Autodesk Inventor part; units mm, degrees
ref_plane "YZ Plane" through (0, 0, 0) normal (1, 0, 0) x (0, 1, 0)
ref_plane "XZ Plane" through (0, 0, 0) normal (0, 1, 0) x (-1, 0, 0)
ref_plane "XY Plane" through (0, 0, 0) normal (0, 0, 1) x (1, 0, 0)
sketch "Skizze1" plane through (0, 0, 0) normal (0, 0, 1) x (1, 0, 0)
  line L0 (-52.5, -10.25) -> (52.5, -10.25)
  line L1 (52.5, -10.25) -> (52.5, 10.25)
  line L2 (52.5, 10.25) -> (-52.5, 10.25)
  line L3 (-52.5, 10.25) -> (-52.5, -10.25)
  line L4 (-52.5, -10.25) -> (52.5, 10.25) construction
  line L5 (52.5, -10.25) -> (-52.5, 10.25) construction
  line L6 (-52.5, 0) -> (52.5, 0) construction
  circle A0 centre (-22.5, 0) radius 2.75
  circle A1 centre (22.5, 0) radius 2.75
  line L7 (0, -14.35) -> (0, 14.35) construction
  point P0 (0, 0)
  dimension "d0" = 105
  dimension "d1" = 20.5
  dimension "d2" = 5.5
  dimension "d3" = 5.5
  dimension "d4" = 45
sketch "Skizze2" plane through (0, 0, 0) normal (1, 0, 0) x (0, 1, 0)
  line L0 (-14.35, 0) -> (14.35, 0) construction
  line L1 (0.25, 0) -> (10.25, 0)
  line L2 (10.25, 0) -> (10.25, 20.5)
  line L3 (10.25, 20.5) -> (0.25, 20.5)
  line L4 (0.25, 20.5) -> (0.25, 0)
  line L5 (0.25, 0) -> (7.85, 0)
  line L6 (7.85, 0) -> (7.85, 18.1)
  line L7 (7.85, 18.1) -> (0.25, 18.1)
  line L8 (0.25, 18.1) -> (0.25, 0)
  point P0 (0, 0)
  point P1 (10.25, 0)
  point P2 (0.25, 18.1)
  dimension "d5" = 20.5
  dimension "d6" = 2.4
  dimension "d7" = 2.4
  dimension "d12" = 10
extrude "Extrusion1" add sketch "Skizze1" against normal blind 1.8
extrude "Extrusion2" add sketch "Skizze2" along normal mid plane 105 contours L6 L7 L4 L3 L2 L1
equation "\"d7\" = d6"
equation "\"d10\" = d0"
properties part number "Door_Handle" material "ABS-Kunststoff"
Here's how the part is built. I have some questions about the finished solid (model axes, mm). A direction names the side the tool comes from. Coordinates: 2 decimals unless noted, no trailing zeros. Write each loop counter-clockwise with the first axis right and the second up, starting at its lowest first coordinate (ties: lowest second). Pieces come first, ordered by that corner, then holes. Notation, with made-up numbers: (50.25, 72.25) - (97.25, 72.25) arc R20 cw to (97.25, 105.25) - close; hole circle Ø2 at (-21.75, -17). An arc over 180 degrees is marked (long way). Use one line per item in the form item = value.
1) Suppose I cut it at C-C, the plane z = 5.5. Write out the boundary of the cut face in (x, y), plus the area to 3 significant figures.
Solved:
outline = (-52.5, 7.85) - (52.5, 7.85) - (52.5, 10.25) - (-52.5, 10.25) - close
area = 252 mm2
2) Thinking about a two-plate mould opening in Z: for faces 1 (the flat face through (-1, 0, -1.8)), 2 (the flat face through (-1, 4, 18.1)), 3 (the flat face through (-1, 0.25, 19)), which applies, released by +Z, released by -Z, zero draft, split by the parting line, or undercut?
Solved:
face_1 = released by -Z
face_2 = undercut
face_3 = zero draft
3) On a 3-axis mill with a long thin cutter (end or side, diameter ignored), from which of +Z, -Z, +X, -X, +Y, -Y can I reach the whole of each face in a straight line? I mean faces 4 (the flat face through (-52.5, 8, 8)), 5 (the flat face through (-1, -1, 0)), 6 (the cylindrical face through (-25.247, 0.121, -0.887)). Say none if no direction works.
Solved:
face_4 = +Z, -Z, -X, +Y, -Y
face_5 = +X, -X, -Y
face_6 = -Z
4) I need wall thicknesses on line 1 (Y direction, x = -22.5, z = -0.8); line 2 (Z direction, x = -27.5, y = 2.25); line 3 (Y direction, x = 33.5, z = 14.25). Which ranges of each line are inside material? Lowest first, please.
Solved:
line_1 = -10.25 to -2.75, 2.75 to 10.25
line_2 = -1.8 to 0, 18.1 to 20.5
line_3 = 7.85 to 10.25
5) Suppose I cut it at D-D, the plane y = -8.5. Write out the boundary of the cut face in (x, z), plus the area to 3 significant figures.
Solved:
outline = (-52.5, -1.8) - (52.5, -1.8) - (52.5, 0) - (-52.5, 0) - close
area = 189 mm2
6) Suppose I cut it at B-B, the plane y = 6.25. Write out the boundary of the cut face in (x, z), plus the area to 3 significant figures.
Solved:
outline = (-52.5, -1.8) - (52.5, -1.8) - (52.5, 0) - (-52.5, 0) - close; (-52.5, 18.1) - (52.5, 18.1) - (52.5, 20.5) - (-52.5, 20.5) - close
area = 441 mm2
7) Suppose I cut it at A-A, the plane x = -22.5. Write out the boundary of the cut face in (y, z).
Solved:
outline = (-10.25, -1.8) - (-2.75, -1.8) - (-2.75, 0) - (-10.25, 0) - close; (0.25, 18.1) - (7.85, 18.1) - (7.85, 0) - (2.75, 0) - (2.75, -1.8) - (10.25, -1.8) - (10.25, 20.5) - (0.25, 20.5) - close
8) I'm going to push flat-ended pins straight in: P1, Ø2, axis at y = -1, z = 18, coming from the +X side; P2, Ø8, axis at x = 17.5, z = 10.5, coming from the -Y side; P3, Ø1.9, axis at x = -13, z = 19.5, coming from the -Y side. Where does each tip first touch, or does it pass through?
Solved:
P1 = through
P2 = 7.85
P3 = 0.25
